```python
from build123d import *

# Parameters (mm, degrees)
F0_R     = 75
F1_DEPTH = 50
F3_DEPTH = 35.5
F5_R     = 52.9296402023
F6_DEPTH = 16


with BuildPart() as f1:
    # F0 (on Top) → F1 (new body)
    with BuildSketch(Plane.XY):
        Circle(F0_R)
    extrude(amount=F1_DEPTH)

    # F2 (on face) → F3 (cut)
    with BuildSketch(Plane(origin=(0, 0, 0), x_dir=(1, 0, 0), z_dir=(0, 0, -1))):
        with BuildLine():
            ThreePointArc((16, -32.2490309932), (30.5941170816, -18.973665961), (36, 0))
            ThreePointArc((36, 0), (30.5941170816, 18.973665961), (16, 32.2490309932))
            Line((16, 32.2490309932), (16, 28.5))
            Line((16, 28.5), (-16, 28.5))
            Line((-16, 28.5), (-16, 32.2490309932))
            ThreePointArc((-16, 32.2490309932), (-36, 0), (-16, -32.2490309932))
            Line((-16, -32.2490309932), (-16, -28.5))
            Line((-16, -28.5), (16, -28.5))
            Line((16, -28.5), (16, -32.2490309932))
        make_face()
        with BuildLine():
            Line((16, 28.5), (16, 32.2490309932))
            ThreePointArc((16, 32.2490309932), (0, 36), (-16, 32.2490309932))
            Line((-16, 32.2490309932), (-16, 28.5))
            Line((-16, 28.5), (16, 28.5))
        make_face()
        with BuildLine():
            ThreePointArc((-16, 32.2490309932), (0, 36), (16, 32.2490309932))
            Line((16, 32.2490309932), (16, 50))
            Line((16, 50), (-16, 50))
            Line((-16, 50), (-16, 32.2490309932))
        make_face()
        with BuildLine():
            Line((16, -50), (16, -32.2490309932))
            ThreePointArc((16, -32.2490309932), (0, -36), (-16, -32.2490309932))
            Line((-16, -32.2490309932), (-16, -50))
            Line((-16, -50), (16, -50))
        make_face()
        with BuildLine():
            ThreePointArc((-16, -32.2490309932), (0, -36), (16, -32.2490309932))
            Line((16, -32.2490309932), (16, -28.5))
            Line((16, -28.5), (-16, -28.5))
            Line((-16, -28.5), (-16, -32.2490309932))
        make_face()
    extrude(amount=-F3_DEPTH, mode=Mode.SUBTRACT)

    # F5 (on offset) → F6 (cut)
    with BuildSketch(Plane.XY.offset(35.5)):
        Circle(F5_R)
    extrude(amount=-F6_DEPTH, mode=Mode.SUBTRACT)


solid = f1.part
```
Could you check a few things on this model? Use its own coordinates, in mm. A direction names the side the tool comes from. Give positions to 0.01 mm unless a question says otherwise; leave off trailing zeros. Loops run counter-clockwise (first coordinate to the right, second up) from the corner with the lowest first, then second, coordinate; pieces in that order, holes last. Notation, with made-up numbers: (-15.5, -36) - (7.5, -36) arc R26 cw to (7.5, 1) - close; hole circle Ø7 at (64, -28.75). An arc over 180 degrees is marked (long way). Answer in a Markdown table with one row per item. Add a question column.
Q1. We'd pull the mould along Z, two halves only. Please class faces 1 (the face through (24.42, -46.96, 27.61)), 2 (the face through (32, 18, 0)), 3 (the face through (-9.764, 74.362, 24.65)): +Z half, -Z half, draft (parallel to the pull), parting line (faces both ways), or undercut.
Q2. Which directions (+Z, -Z, +X, -X, +Y, -Y) give clear straight access to the entire face, cutting with the end or side of a thin tool? Please do faces 4 (the face through (16, 41, 10)), 5 (the face through (23, 28, 19.5)), 6 (the face through (-1, 1, 50)).
Q3. If we section it at B-B (x = 0): List the corners of the cut face in (y, z) for me.
Q4. If we section it at C-C (x = 40): List the corners of the cut face in (y, z) for me, plus the area to 3 significant figures.
Q5. For pin 1 (12 mm diameter, centred on y = -38.5, z = 38.5, fed in from -X); pin 2 (15.5 mm diameter, centred on x = 2, z = 12.5, fed in from +Y); pin 3 (10 mm diameter, centred on x = -6, z = 35, fed in from -Y), each with a flat end and sliding along its axis, tell me the tip position at first contact or that it passes through.
Q6. If we section it at D-D (y = -7): List the corners of the cut face in (x, z) for me, plus the area to 3 significant figures.
Q7. If we section it at A-A (z = 17.5): List the corners of the cut face in (x, y) for me.
Q8. Please list where these lines run through material, in increasing order: L1, parallel to Y at x = 0, z = 31; L2, parallel to Z at x = 32, y = -40; L3, parallel to Z at x = 7.5, y = 15.5. Write a range as from..to.
The answers:
| question | item | result |
|---|---|---|
| 1 | face 1 | undercut |
| 1 | face 2 | -Z half |
| 1 | face 3 | draft |
| 2 | face 4 | -Z |
| 2 | face 5 | none |
| 2 | face 6 | +Z, +X, -X, +Y, -Y |
| 3 | outline | (-75, 0) - (-50, 0) - (-50, 19.5) - (-52.93, 19.5) - (-52.93, 35.5) - (52.93, 35.5) - (52.93, 19.5) - (50, 19.5) - (50, 0) - (75, 0) - (75, 50) - (-75, 50) - close |
| 4 | outline | (-63.44, 0) - (63.44, 0) - (63.44, 50) - (-63.44, 50) - close; hole (-34.66, 19.5) - (34.66, 19.5) - (34.66, 35.5) - (-34.66, 35.5) - close |
| 4 | area | 5,240 mm^2 |
| 5 | pin 1 | stops at x = -67.59 |
| 5 | pin 2 | stops at y = 75 |
| 5 | pin 3 | stops at y = -74.99 |
| 6 | outline | (-74.67, 0) - (-35.31, 0) - (-35.31, 19.5) - (-52.46, 19.5) - (-52.46, 35.5) - (52.46, 35.5) - (52.46, 19.5) - (35.31, 19.5) - (35.31, 0) - (74.67, 0) - (74.67, 50) - (-74.67, 50) - close |
| 6 | area | 4,410 mm^2 |
| 7 | outline | circle Ø150 at (0, 0); hole (-16, -50) - (16, -50) - (16, -32.25) arc R36 ccw to (16, 32.25) - (16, 50) - (-16, 50) - (-16, 32.25) arc R36 ccw to (-16, -32.25) - close |
| 8 | L1 | y = -75..-52.93, 52.93..75 |
| 8 | L2 | z = 0..19.5, 35.5..50 |
| 8 | L3 | z = 35.5..50 |
